```python
from build123d import *

# Parameters (mm, degrees)
SKETCH1_R           = 16
SKETCH1_R_2         = 14
BOSS_EXTRUDE1_DEPTH = 10
BOSS_EXTRUDE2_DEPTH = 4
BOSS_EXTRUDE3_DEPTH = 14
SKETCH4_R           = 18
BOSS_EXTRUDE4_DEPTH = 4
SKETCH5_R           = 18
SKETCH5_R_2         = 16
BOSS_EXTRUDE5_DEPTH = 8


with BuildPart() as part:
    # Sketch1 → Boss-Extrude1 (new body)
    with BuildSketch(Plane(origin=(0, 0, 0), x_dir=(0, 0, -1), z_dir=(1, 0, 0))):
        Circle(SKETCH1_R)
        Circle(SKETCH1_R_2, mode=Mode.SUBTRACT)
    extrude(amount=-BOSS_EXTRUDE1_DEPTH)

    # Sketch2 → Boss-Extrude2 (add)
    with BuildSketch(Plane(origin=(0, 0, 0), x_dir=(0, 0, -1), z_dir=(1, 0, 0))):
        with BuildLine():
            Line((-7, 14.288943502), (-7, 20))
            Line((-7, 20), (7, 20))
            Line((7, 20), (7, 14.288943502))
            ThreePointArc((7, 14.288943502), (0, -15.911439483), (-7, 14.288943502))
        make_face()
    extrude(amount=BOSS_EXTRUDE2_DEPTH)

    # Sketch3 → Boss-Extrude3 (add)
    with BuildSketch(Plane(origin=(0, 0, -7), x_dir=(-1, 0, 0), z_dir=(0, 0, -1))):
        with BuildLine():
            Line((0, 20), (-4, 20))
            Line((-4, 20), (-4, 30))
            ThreePointArc((-4, 30), (-2.828427125, 32.828427125), (0, 34))
            Line((0, 34), (38, 34))
            Line((38, 34), (38, 30))
            Line((38, 30), (4, 30))
            ThreePointArc((4, 30), (1.171572875, 28.828427125), (0, 26))
            Line((0, 26), (0, 20))
        make_face()
    extrude(amount=-BOSS_EXTRUDE3_DEPTH)

    # Sketch4 → Boss-Extrude4 (add)
    with BuildSketch(Plane(origin=(0, 34, 0), x_dir=(1, 0, 0), z_dir=(0, 1, 0))):
        with Locations((-38, 0)):
            Circle(SKETCH4_R)
    extrude(amount=-BOSS_EXTRUDE4_DEPTH)

    # Sketch5 → Boss-Extrude5 (add)
    with BuildSketch(Plane(origin=(0, 34, 0), x_dir=(1, 0, 0), z_dir=(0, 1, 0))):
        with Locations((-38, 0)):
            Circle(SKETCH5_R)
        with Locations((-38, 0)):
            Circle(SKETCH5_R_2, mode=Mode.SUBTRACT)
    extrude(amount=BOSS_EXTRUDE5_DEPTH)


solid = part.part
```
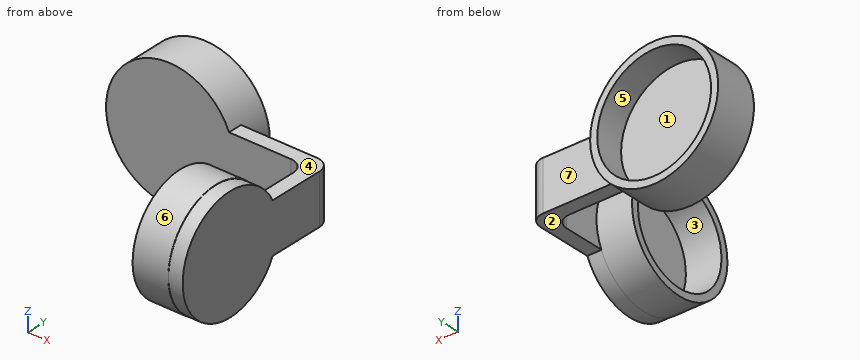
Design review of the part built by this model. Coordinates are the model's own, in mm. Face numbers are marked on the shaded views. A direction names the side the tool comes from. Round coordinates to 2 decimals unless told otherwise and drop trailing zeros. Write each loop counter-clockwise with the first axis right and the second up, starting at its lowest first coordinate (ties: lowest second). Pieces come first, ordered by that corner, then holes. Notation, with made-up numbers: (37.25, 81.5) -> (72.25, 81.5) arc R22 ccw to (72.25, 95.5) -> close; hole circle Ø11 at (14.5, 79). An arc over 180 degrees is marked (long way). Write item = value, one per line. Start each with the question number.
1) Clearance check with flat-ended pins moving along their axes: pin 1 (6 mm diameter, centred on x = -11.5, y = 25, fed in from -Z); pin 2 (6 mm diameter, centred on x = -37.5, z = -7, fed in from -Y); pin 3 (5 mm diameter, centred on y = -10, z = 3, fed in from -X); pin 4 (13 mm diameter, centred on y = 18, z = 0.5, fed in from -X). State where each tip first meets the part, or that it passes through.
2) Take a section at B-B, the plane x = -38. State the section outline as (y, z) points.
3) Take a section at C-C, the plane z = 0. State the section outline as (x, y) points.
4) Take a section at A-A, the plane z = 13. State the section outline as (x, y) points.
5) Mouldability with a two-part tool opening along Z and no side actions: class the marked faces 5, 6 and 7 as +Z half, -Z half, draft (parallel to the pull), parting line (faces both ways), or undercut.
6) Take a section at D-D, the plane y = 0. State the section outline as (x, z) points.
7) Wall thickness on probe 1 along Y at (x, z) = (-4, 0); probe 2 along Z at (x, y) = (-38, 37); probe 3 along X at (y, z) = (5.5, 10): over which ranges is each line inside the solid? List them lowest first. Write a range as from..to.
8) Tool access review of the marked faces 1, 2, 3 and 4: name each direction out of +Z, -Z, +X, -X, +Y, -Y from which nothing blocks a thin tool from reaching the whole face with its end or side.
Results list:
q1.pin_1 = through
q1.pin_2 = 30
q1.pin_3 = 0
q1.pin_4 = -10
q2.outline = (30, -18) -> (42, -18) -> (42, -16) -> (34, -16) -> (34, 16) -> (42, 16) -> (42, 18) -> (30, 18) -> close
q3.outline = (-56, 30) -> (-4, 30) arc R4 cw to (0, 26) -> (0, 16) -> (-10, 16) -> (-10, 14) -> (0, 14) -> (0, -14) -> (-10, -14) -> (-10, -16) -> (0, -16) -> (0, -15.91) -> (4, -15.91) -> (4, 30) arc R4 ccw to (0, 34) -> (-20, 34) -> (-20, 42) -> (-22, 42) -> (-22, 34) -> (-54, 34) -> (-54, 42) -> (-56, 42) -> close
q4.outline = (-50.45, 30) -> (-25.55, 30) -> (-25.55, 42) -> (-28.67, 42) -> (-28.67, 34) -> (-47.33, 34) -> (-47.33, 42) -> (-50.45, 42) -> close; (-10, -9.33) -> (0, -9.33) -> (0, -9.17) -> (4, -9.17) -> (4, 9.17) -> (0, 9.17) -> (0, 9.33) -> (-10, 9.33) -> (-10, 5.2) -> (0, 5.2) -> (0, -5.2) -> (-10, -5.2) -> close
q5.face_5 = undercut
q5.face_6 = parting line
q5.face_7 = draft
q6.outline = (-10, -16) -> (0, -16) -> (0, -15.91) -> (4, -15.91) -> (4, 15.91) -> (0, 15.91) -> (0, 16) -> (-10, 16) -> (-10, 14) -> (0, 14) -> (0, -14) -> (-10, -14) -> close
q7.probe_1 = -16..-14, 14..16, 30..34
q7.probe_2 = -18..-16, 16..18
q7.probe_3 = 0..4
q8.face_1 = +Y
q8.face_2 = -Z, +X, +Y
q8.face_3 = -X
q8.face_4 = +Z, +X, +Y
